```python
from build123d import *

# Parameters (mm, degrees)
BOSS_EXTRUDE1_DEPTH = 50
BOSS_EXTRUDE4_DEPTH = 50
SKETCH5_W           = 50
SKETCH5_H           = 20
CUT_EXTRUDE2_DEPTH  = 50
SKETCH6_W           = 50
SKETCH6_H           = 20
CUT_EXTRUDE3_DEPTH  = 50
SKETCH7_R           = 10
CUT_EXTRUDE4_DEPTH  = 50
SKETCH8_R           = 10
CUT_EXTRUDE5_DEPTH  = 50


with BuildPart() as part:
    # Sketch2 → Boss-Extrude1 (new body)
    with BuildSketch(Plane(origin=(0, 0, 0), x_dir=(1, 0, 0), z_dir=(0, 1, 0))):
        with BuildLine():
            Line((-60, 25), (65, 25))
            ThreePointArc((65, 25), (90, 0), (65, -25))
            Line((65, -25), (-60, -25))
            Line((-60, -25), (-60, 25))
        make_face()
    extrude(amount=BOSS_EXTRUDE1_DEPTH)

    # Sketch3 → Boss-Extrude4 (add)
    with BuildSketch(Plane.XY.offset(25)):
        with BuildLine():
            Line((-60, 50), (-60, 0))
            ThreePointArc((-60, 0), (-85, 25), (-60, 50))
        make_face()
    extrude(amount=-BOSS_EXTRUDE4_DEPTH)

    # Sketch5 → Cut-Extrude2 (cut)
    with BuildSketch(Plane(origin=(0, 50, 0), x_dir=(1, 0, 0), z_dir=(0, 1, 0))):
        with Locations((-60, 0)):
            Rectangle(SKETCH5_W, SKETCH5_H)
    extrude(amount=-CUT_EXTRUDE2_DEPTH, mode=Mode.SUBTRACT)

    # Sketch6 → Cut-Extrude3 (cut)
    with BuildSketch(Plane.XY.offset(25)):
        with Locations((65, 25)):
            Rectangle(SKETCH6_W, SKETCH6_H)
    extrude(amount=-CUT_EXTRUDE3_DEPTH, mode=Mode.SUBTRACT)

    # Sketch7 → Cut-Extrude4 (cut)
    with BuildSketch(Plane(origin=(0, 50, 0), x_dir=(1, 0, 0), z_dir=(0, 1, 0))):
        with Locations((65, 0)):
            Circle(SKETCH7_R)
    extrude(amount=-CUT_EXTRUDE4_DEPTH, mode=Mode.SUBTRACT)

    # Sketch8 → Cut-Extrude5 (cut)
    with BuildSketch(Plane(origin=(0, 0, -25), x_dir=(-1, 0, 0), z_dir=(0, 0, -1))):
        with Locations((60, 25)):
            Circle(SKETCH8_R)
    extrude(amount=-CUT_EXTRUDE5_DEPTH, mode=Mode.SUBTRACT)


solid = part.part
```
Could you check a few things on this model? Use its own coordinates, in mm. A direction names the side the tool comes from. Round coordinates to 2 decimals unless told otherwise and drop trailing zeros. Write each loop counter-clockwise with the first axis right and the second up, starting at its lowest first coordinate (ties: lowest second). Pieces come first, ordered by that corner, then holes.
(1) Suppose I cut it at B-B on y = 25. Write out the boundary of the cut face in (x, z), and give its area (3 significant figures).
Findings below:
outline: (-85, -25) - (-70, -25) - (-70, -10) - (-85, -10) - close; (-85, 10) - (-70, 10) - (-70, 25) - (-85, 25) - close; (-50, -25) - (40, -25) - (40, 25) - (-50, 25) - (-50, 10) - (-35, 10) - (-35, -10) - (-50, -10) - close
area: 4,650 mm2
(2) Suppose I cut it at A-A on z = 0. Write out the boundary of the cut face in (x, y).
Findings below:
outline: (-35, 0) - (55, 0) - (55, 15) - (40, 15) - (40, 35) - (55, 35) - (55, 50) - (-35, 50) - close; (75, 0) - (90, 0) - (90, 15) - (75, 15) - close; (75, 35) - (90, 35) - (90, 50) - (75, 50) - close
(3) If I drill on probe 1 along Z at (x, y) = (65, 6); probe 2 along Y at (x, z) = (42, -3); probe 3 along X at (y, z) = (38, 0), over which ranges is the centre line in solid material (lowest first)?
Findings below:
probe 1: z = -25 to -10, 10 to 25
probe 2: y = 0 to 15, 35 to 50
probe 3: x = -35 to 55, 75 to 90
(4) Suppose I cut it at C-C on z = -20. Write out the boundary of the cut face in (x, y), and give its area (3 significant figures).
Findings below:
outline: (-60, 0) - (80, 0) - (80, 15) - (40, 15) - (40, 35) - (80, 35) - (80, 50) - (-60, 50) arc R25 ccw to start; hole circle Ø20 at (-60, 25)
area: 6,870 mm2
(5) Thinking about a two-plate mould opening in X: for faces 4 (the face through (55, 8, 0)), 5 (the face through (54, 15, 0)), 6 (the face through (89.994, 7.395, -0.55)), which applies, +X half, -X half, draft (parallel to the pull), parting line (faces both ways), or undercut?
Findings below:
face 4: undercut
face 5: draft
face 6: +X half
(6) Suppose I cut it at D-D on x = -63.5. Write out the boundary of the cut face in (y, z), and give its area (3 significant figures).
Findings below:
outline: (0.25, -25) - (15.63, -25) - (15.63, -10) - (0.25, -10) - close; (0.25, 10) - (15.63, 10) - (15.63, 25) - (0.25, 25) - close; (34.37, -25) - (49.75, -25) - (49.75, -10) - (34.37, -10) - close; (34.37, 10) - (49.75, 10) - (49.75, 25) - (34.37, 25) - close
area: 923 mm2
(7) Which directions (+Z, -Z, +X, -X, +Y, -Y) give clear straight access to the entire face, cutting with the end or side of a thin tool? Please do faces 1 (the face through (-49, 25, -10)), 2 (the face through (16, 0, 0)), 3 (the face through (40, 25, 0)).
Findings below:
face 1: -X, +Y, -Y
face 2: +Z, -Z, +X, -X, -Y
face 3: +Z, -Z, +X
(8) For pin 1 (16 mm diameter, centred on y = 25.5, z = 10.5, fed in from +X); pin 2 (6 mm diameter, centred on y = 16.5, z = -9, fed in from +X); pin 3 (5 mm diameter, centred on y = 26.5, z = 8, fed in from -X), each with a flat end and sliding along its axis, tell me the tip position at first contact or that it passes through.
Findings below:
pin 1: stops at x = 40
pin 2: stops at x = 89.17
pin 3: stops at x = -85
